Input: part model. Units: mm. Frame: model coordinates. Round coordinates to 2 decimals unless told otherwise and drop trailing zeros. Order: outer loops, then holes, each group sorted by start corner. A loop starts at its lowest first (then second) coordinate and runs counter-clockwise, first axis right, second up. Notation, with made-up numbers: (5, -28) -> (34, -28) arc R25 ccw to (34, -14) -> close; hole circle Ø1 at (25, -30). An arc over 180 degrees is marked (long way). Use a Markdown table: item, result.
Autodesk Inventor part; units mm, degrees
ref_plane "YZ Plane" through (0, 0, 0) normal (1, 0, 0) x (0, 1, 0)
ref_plane "XZ Plane" through (0, 0, 0) normal (0, 1, 0) x (-1, 0, 0)
ref_plane "XY Plane" through (0, 0, 0) normal (0, 0, 1) x (1, 0, 0)
sketch "Sketch1" plane through (0, 0, 0) normal (0, 1, 0) x (-1, 0, 0)
  line L0 (45, 0) -> (0, 0)
  line L1 (0, 0) -> (0, -300)
  line L2 (0, -300) -> (45, -300)
  line L3 (45, -300) -> (45, 0)
  circle A0 centre (22.5, -22.5) radius 5
  circle A1 centre (22.5, -277.5) radius 5
  line L4 (79.2183, -150) -> (-46.459, -150) construction
  circle A2 centre (22.5, -121.5) radius 4.8
  circle A3 centre (22.5, -178.5) radius 4.8
  dimension "d0" = 300
  dimension "d1" = 45
  dimension "d2" = 10
  dimension "d3" = 10
  dimension "d4" = 22.5
  dimension "d5" = 22.5
  dimension "d6" = 22.5
  dimension "d7" = 22.5
  dimension "d8" = 150
  dimension "d9" = 9.6
  dimension "d10" = 28.5
  dimension "d11" = 22.5
  dimension "d12" = 22.5
  dimension "d13" = 28.5
extrude "Extrusion1" add sketch "Sketch1" along normal blind 10
properties part number "1211_Distal Roller Plate_V1" material "Wood (Birch)"
1) Cut plane D-D on z = -277.5. Return loops of the section in (x, y).
Results found:
| item | result |
|---|---|
| outline | (-45, 0) -> (-27.5, 0) -> (-27.5, 10) -> (-45, 10) -> close; (-17.5, 0) -> (0, 0) -> (0, 10) -> (-17.5, 10) -> close |
2) Cut plane B-B on z = -178.5. Return loops of the section in (x, y), and give its area (3 significant figures).
Results found:
| item | result |
|---|---|
| outline | (-45, 0) -> (-27.3, 0) -> (-27.3, 10) -> (-45, 10) -> close; (-17.7, 0) -> (0, 0) -> (0, 10) -> (-17.7, 10) -> close |
| area | 354 mm² |
3) Cut plane A-A on x = -22.5. Return loops of the section in (y, z), and give its area (3 significant figures).
Results found:
| item | result |
|---|---|
| outline | (0, -300) -> (10, -300) -> (10, -282.5) -> (0, -282.5) -> close; (0, -272.5) -> (10, -272.5) -> (10, -183.3) -> (0, -183.3) -> close; (0, -173.7) -> (10, -173.7) -> (10, -126.3) -> (0, -126.3) -> close; (0, -116.7) -> (10, -116.7) -> (10, -27.5) -> (0, -27.5) -> close; (0, -17.5) -> (10, -17.5) -> (10, 0) -> (0, 0) -> close |
| area | 2,610 mm² |
4) Line query: L1, parallel to Z at x = -22.5, y = 2.5; L2, parallel to X at y = 6, z = -277.5; L3, parallel to Z at x = -26, y = 6.5. Output: solid intervals per line, ascending. Write a range as [from, to].
Results found:
| item | result |
|---|---|
| L1 | z = [-300, -282.5], [-272.5, -183.3], [-173.7, -126.3], [-116.7, -27.5], [-17.5, 0] |
| L2 | x = [-45, -27.5], [-17.5, 0] |
| L3 | z = [-300, -281.07], [-273.93, -181.78], [-175.22, -124.78], [-118.22, -26.07], [-18.93, 0] |
5) Pull-direction query (X, two-part tool) for faces 1 (the flat face through (-22, 5, -300)), 2 (the cylindrical face through (-21.849, 4.93, -282.457)), 3 (the cylindrical face through (-21.42, 4.93, -17.62)), 4 (the flat face through (0, 5, -148)); classes: +X half, -X half, draft (parallel to the pull), parting line (faces both ways), or undercut.
Results found:
| item | result |
|---|---|
| face 1 | draft |
| face 2 | undercut |
| face 3 | undercut |
| face 4 | +X half |
6) Cut plane C-C on y = 5.5. Return loops of the section in (x, z).
Results found:
| item | result |
|---|---|
| outline | (-45, -300) -> (0, -300) -> (0, 0) -> (-45, 0) -> close; hole circle Ø10 at (-22.5, -277.5); hole circle Ø10 at (-22.5, -22.5); hole circle Ø9.6 at (-22.5, -178.5); hole circle Ø9.6 at (-22.5, -121.5) |
